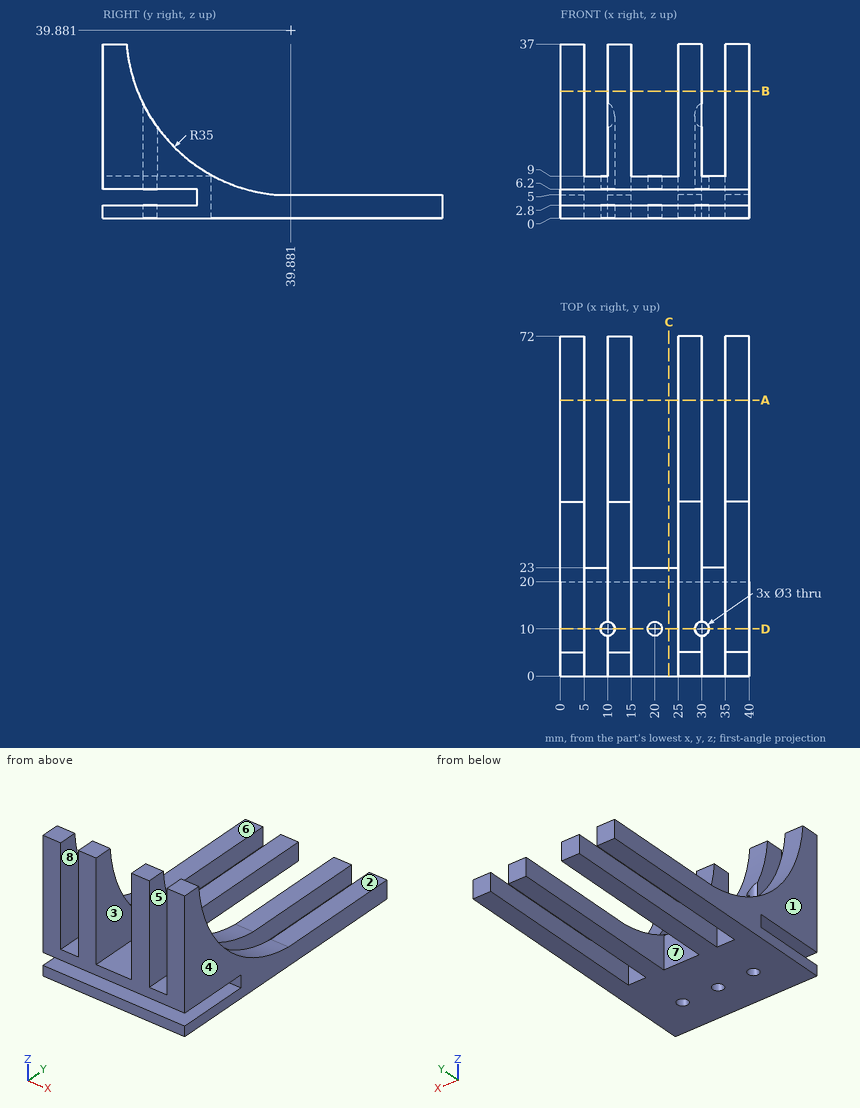
Drawing for the job (mm, zero at the part's lowest x, y, z). A direction names the side the tool comes from. Give positions to 0.01 mm unless a question says otherwise; leave off trailing zeros. Write each loop counter-clockwise with the first axis right and the second up, starting at its lowest first coordinate (ties: lowest second). Pieces come first, ordered by that corner, then holes. Notation, with made-up numbers: (-22, -15.75) -> (20, -15.75) arc R18 ccw to (20, 0.25) -> close; hole circle Ø1 at (-10, -40). An arc over 180 degrees is marked (long way). Put each result on its own line as item: value. Start each with the question number.
Item 1: Pin check, flat tips, straight feed: pin 1 Ø5.5 at (x, y) = (32, 13) entering from +Z; pin 2 Ø12 at (x, z) = (25, 29) entering from -Y; pin 3 Ø4 at (x, y) = (10, 10) entering from +Z; pin 4 Ø6 at (x, z) = (12, 17) entering from +Y. Stop position of each tip, or through.
Item 2: Cut at C-C (x = 23). List the corners of the cut face in (y, z).
Item 3: Cut at D-D (y = 10). State how many separate pieces and enclosed holes the cut face has, then the cut area to 3 significant figures.
Item 4: Which spindle directions (+Z, -Z, +X, -X, +Y, -Y) get a long thin tool onto all of the face, cutting with end or side? Do the marked faces 5, 6, 7 and 8. Say none if no direction does.
Item 5: Cut at B-B (z = 27). List the corners of the cut face in (x, y).
Item 6: Pull direction X, two halves, no side cores. Call the marked faces 1, 2, 3 and 4: pulls with the +X half, pulls with the -X half, needs draft (parallel to the pull), parting line crosses it, or undercut.
Item 7: Wall check: L1, parallel to X at y = 10, z = 16; L2, parallel to X at y = 18, z = 10.5; L3, parallel to Z at x = 33, y = 18.5. Give the ranges that are in metal, low to high. Write a range as [from, to].
Item 8: Cut at A-A (y = 58.5). List the corners of the cut face in (x, z), then the cut area to 3 significant figures.
Answer list:
1. pin 1: stops at z = 19.44
1. pin 2: stops at y = 0
1. pin 3: stops at z = 25.44
1. pin 4: stops at y = 16.32
2. outline: (0, 0) -> (23, 0) -> (23, 9) -> (0, 9) -> (0, 6.2) -> (20, 6.2) -> (20, 2.8) -> (0, 2.8) -> close
3. separate pieces: 8
3. enclosed holes: 0
3. area: 389 mm2
4. face 5: +Z, +Y, -Y
4. face 6: +Z, +X, -X, +Y
4. face 7: +Z, -Z, +Y
4. face 8: +Z, +Y
5. outline: (0, 0) -> (5, 0) -> (5, 7.34) -> (0, 7.34) -> close; (10, 0) -> (15, 0) -> (15, 7.34) -> (10, 7.34) -> close; (25, 0) -> (30, 0) -> (30, 7.34) -> (25, 7.34) -> close; (35, 0) -> (40, 0) -> (40, 7.34) -> (35, 7.34) -> close
6. face 1: pulls with the -X half
6. face 2: needs draft
6. face 3: undercut
6. face 4: pulls with the +X half
7. L1: x = [0, 5], [11.5, 15], [25, 28.5], [35, 40]
7. L2: x = [0, 5], [10, 15], [25, 30], [35, 40]
7. L3: z = [0, 2.8], [6.2, 9]
8. outline: (0, 0) -> (5, 0) -> (5, 5) -> (0, 5) -> close; (10, 0) -> (15, 0) -> (15, 5) -> (10, 5) -> close; (25, 0) -> (30, 0) -> (30, 5) -> (25, 5) -> close; (35, 0) -> (40, 0) -> (40, 5) -> (35, 5) -> close
8. area: 100 mm2
